Source: three-view drawing plus pictorial views. Frame: mm from the lowest corner of the part. A direction names the side the tool comes from. Coordinates: 2 decimals unless noted, no trailing zeros. Write each loop counter-clockwise with the first axis right and the second up, starting at its lowest first coordinate (ties: lowest second). Pieces come first, ordered by that corner, then holes. Notation, with made-up numbers: (20.5, -20.5) -> (61.5, -20.5) arc R35 cw to (61.5, 17.5) -> close; hole circle Ø6 at (44, 56.25). An arc over 180 degrees is marked (long way). One line per question, with ' | ' between items. Start each with the question number.
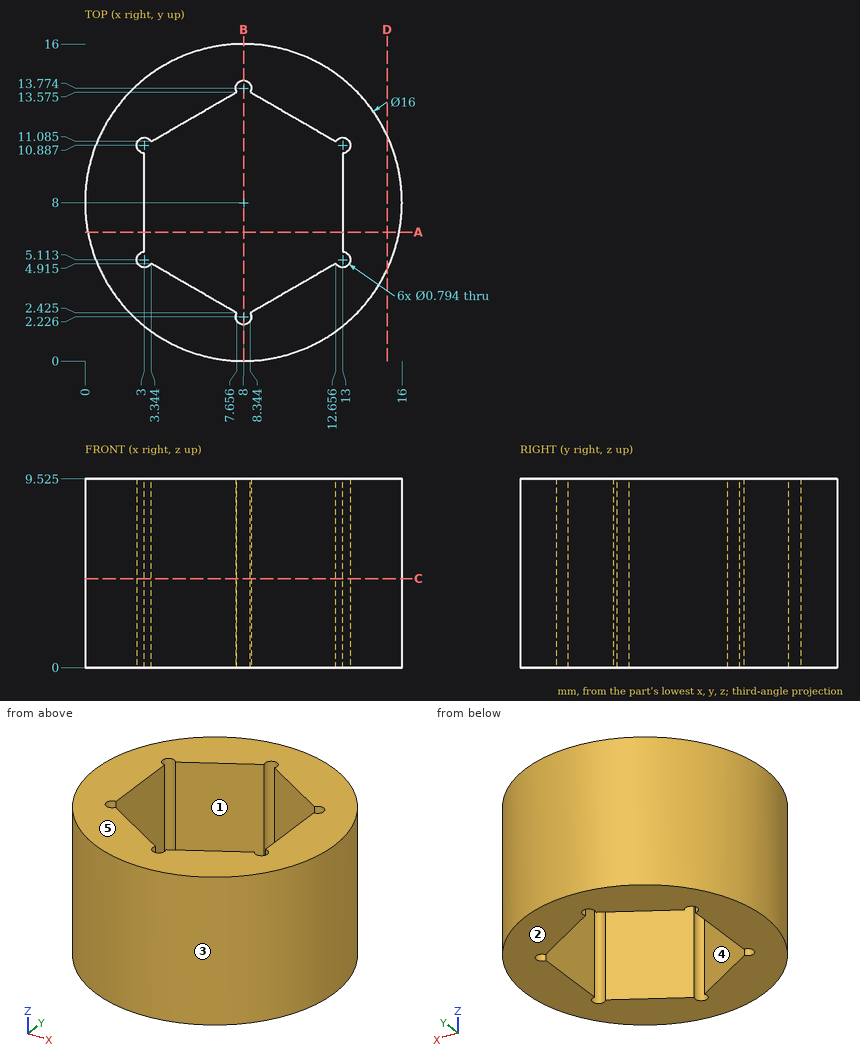
1) Section B-B, the plane x = 8. Return loops of the section in (y, z) (1 decimal).
2) Pull-direction query (Y, two-part tool) for the marked faces 1, 2 and 3; classes: released by +Y, released by -Y, zero draft, split by the parting line, or undercut.
3) Access query for the marked faces 4 and 5. Directions: +Z, -Z, +X, -X, +Y, -Y. A direction counts if a zero-diameter tool reaches every point of the face in a straight line with its end or side. Return the directions, or none.
4) Ray query, line 1 (Y direction, x = 8, z = 3.75); line 2 (Y direction, x = 12.5, z = 5) (1 decimal); line 3 (X direction, y = 13, z = 5) (1 decimal). Return the intervals inside material, ascending.
5) Section D-D, the plane x = 15.25. Return loops of the section in (y, z) (1 decimal).
6) First-contact query: P1, Ø3, axis at x = 5, z = 2.5, coming from the +Y side; P2, Ø4, axis at x = 5.5, z = 3.5, coming from the -Y side; P3, Ø5, axis at y = 13.5, z = 7, coming from the +X side. Flat tips, straight axial feed; report the tip coordinate or a pass-through.
7) Section C-C, the plane z = 4.5. Return loops of the section in (x, y) (1 decimal).
8) Section A-A, the plane y = 6.5. Return loops of the section in (x, z) (1 decimal).
Answer block:
1) outline: (0, 0) -> (1.8, 0) -> (1.8, 9.5) -> (0, 9.5) -> close; (14.2, 0) -> (16, 0) -> (16, 9.5) -> (14.2, 9.5) -> close
2) face 1: undercut | face 2: zero draft | face 3: split by the parting line
3) face 4: +Z, -Z | face 5: +Z, +X, -X, +Y, -Y
4) line 1: y = 0 to 1.83, 14.17 to 16 | line 2: y = 1.4 to 4.8, 11.2 to 14.6 | line 3: x = 1.8 to 6.7, 9.3 to 14.2
5) outline: (4.6, 0) -> (11.4, 0) -> (11.4, 9.5) -> (4.6, 9.5) -> close
6) P1: stops at y = 15.86 | P2: stops at y = 0.02 | P3: stops at x = 15.42
7) outline: circle Ø16 at (8, 8); hole (3, 5.5) arc R0.4 ccw (long way) to (3.3, 4.9) -> (7.7, 2.4) arc R0.4 ccw (long way) to (8.3, 2.4) -> (12.7, 4.9) arc R0.4 ccw (long way) to (13, 5.5) -> (13, 10.5) arc R0.4 ccw (long way) to (12.7, 11.1) -> (8.3, 13.6) arc R0.4 ccw (long way) to (7.7, 13.6) -> (3.3, 11.1) arc R0.4 ccw (long way) to (3, 10.5) -> close
8) outline: (0.1, 0) -> (3, 0) -> (3, 9.5) -> (0.1, 9.5) -> close; (13, 0) -> (15.9, 0) -> (15.9, 9.5) -> (13, 9.5) -> close
